Check sheet for the modelled part. Datum: model origin and axes. Units: mm. Coordinates: 2 decimals unless noted, no trailing zeros. Loops run counter-clockwise (first coordinate to the right, second up) from the corner with the lowest first, then second, coordinate; pieces in that order, holes last.
```python
from build123d import *

# Parameters (mm, degrees)
F1_DEPTH = 20
F3_DEPTH = 2635
F5_DEPTH = 20
F6_R     = 5


with BuildPart() as f1:
    # F0 (on Top) → F1 (new body)
    with BuildSketch(Plane.XY):
        Polygon((-19.75, -17.750001), (-19.75, -19.75), (-13.75, -19.75), (19.75, 13.75), (19.75, 19.75), (17.750001, 19.75), (17.750001, 14.578427), (-14.578427, -17.750001), align=None)
    extrude(amount=F1_DEPTH)

    # F2 (on face) → F3 (join)
    with BuildSketch(Plane.XY.offset(20)):
        Polygon((-19.75, -19.75), (-13.75, -19.75), (19.75, 13.75), (19.75, 19.75), (11.25, 19.75), (11.25, 23.75), (7.25, 27.75), (7.25, 24.921573), (9.25, 22.921573), (9.25, 19.75), (9.25, 17.750001), (17.750001, 17.750001), (17.750001, 14.578427), (14.335787, 11.164213), (-11.164213, -14.335787), (-14.578427, -17.750001), (-17.750001, -17.750001), (-17.750001, -9.25), (-19.75, -9.25), (-22.921573, -9.25), (-24.921573, -7.25), (-27.75, -7.25), (-23.75, -11.25), (-19.75, -11.25), align=None)
    extrude(amount=F3_DEPTH)

    # F4 (on face) → F5 (join)
    with BuildSketch(Plane.XY.offset(2655)):
        Polygon((19.75, 13.75), (19.75, 19.75), (17.750001, 19.75), (17.750001, 14.578427), (-14.578427, -17.750001), (-19.75, -17.750001), (-19.75, -19.75), (-13.75, -19.75), align=None)
    extrude(amount=F5_DEPTH)

    # F6
    f6_edges = [f1.edges().sort_by_distance(p)[0] for p in [
        (19.75, 13.75, 1337.5),
        (-13.75, -19.75, 1337.5),
    ]]
    fillet(f6_edges, radius=F6_R)


solid = f1.part
```
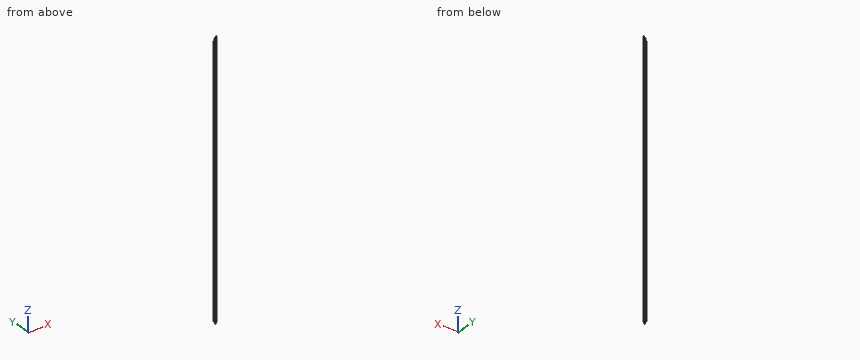
1) Scan lines: line 1 (Y direction, x = -21, z = 172); line 2 (Y direction, x = -16, z = 1572); line 3 (X direction, y = -8, z = 1097.5). Record each from-to range of solid material in increasing order.
Answer sheet:
line 1: y = -11.25 to -9.25
line 2: y = -19.75 to -17.75
line 3: x = -27 to -24.17, -4.83 to -2
2) Section check B-B on y = 1.5. Enter the section's corners in (x, z), plus the area to 3 significant figures.
Answer sheet:
outline: (4.67, 0) - (7.5, 0) - (7.5, 2675) - (4.67, 2675) - close
area: 7,570 mm2
3) Section check C-C on x = -4.5. Enter the section's corners in (y, z).
Answer sheet:
outline: (-10.5, 0) - (-7.67, 0) - (-7.67, 2675) - (-10.5, 2675) - close
4) Section check A-A on z = 746. Enter the section's corners in (x, y).
Answer sheet:
outline: (-27.75, -7.25) - (-23.75, -11.25) - (-19.75, -11.25) - (-19.75, -19.75) - (-15.82, -19.75) arc R5 ccw to (-12.29, -18.29) - (18.29, 12.29) arc R5 ccw to (19.75, 15.82) - (19.75, 19.75) - (11.25, 19.75) - (11.25, 23.75) - (7.25, 27.75) - (7.25, 24.92) - (9.25, 22.92) - (9.25, 17.75) - (17.75, 17.75) - (17.75, 14.58) - (-14.58, -17.75) - (-17.75, -17.75) - (-17.75, -9.25) - (-22.92, -9.25) - (-24.92, -7.25) - close
5) Depth check by flat-ended pin: pin 1 (4 mm diameter, centred on x = -21.5, z = 2238, fed in from +Y); pin 2 (4 mm diameter, centred on y = 8.5, z = 631.5, fed in from +X); pin 3 (2.5 mm diameter, centred on y = 19.5, z = 1461, fed in from -X); pin 4 (5 mm diameter, centred on x = -24.5, y = -15, fed in from -Z). Enter the tip coordinate at first touch or a pass-through.
Answer sheet:
pin 1: stops at y = -8.67
pin 2: stops at x = 16.5
pin 3: stops at x = 9.25
pin 4: passes through
